The listing builds one solid part. Answer for the finished solid, in the listing's coordinates (mm). A direction names the side the tool comes from. Give positions to 0.01 mm unless a question says otherwise; leave off trailing zeros. Order: outer loops, then holes, each group sorted by start corner. A loop starts at its lowest first (then second) coordinate and runs counter-clockwise, first axis right, second up.
Autodesk Inventor part; units mm, degrees
ref_plane "YZ Plane" through (0, 0, 0) normal (1, 0, 0) x (0, 1, 0)
ref_plane "XZ Plane" through (0, 0, 0) normal (0, 1, 0) x (-1, 0, 0)
ref_plane "XY Plane" through (0, 0, 0) normal (0, 0, 1) x (1, 0, 0)
sketch "Sketch1" plane through (0, 0, 0) normal (0, 0, 1) x (1, 0, 0)
  line L0 (-33, 0) -> (33, 0)
  line L1 (33, 0) -> (33, -58)
  line L2 (33, -58) -> (-33, -58)
  line L3 (-33, -58) -> (-33, 0)
  point P0 (0, 0)
  dimension "d0" = 58
  dimension "d1" = 66
  dimension "d2" = 33
  dimension "d3" = 0
extrude "clamp_base" add sketch "Sketch1" against normal blind 190
sketch "Sketch2" plane through (0, 0, 0) normal (0, 0, 1) x (1, 0, 0)
  line L0 (-25, -58) -> (25, -58)
  line L1 (25, -58) -> (25, -8)
  line L2 (25, -8) -> (-25, -8)
  line L3 (-25, -8) -> (-25, -58)
  line L4 (-33, -58) -> (33, -58)
  point P0 (0, 0)
  dimension "d6" = 50
  dimension "d7" = 50
  dimension "d8" = 25
extrude "clamp_extrusion" cut sketch "Sketch2" against normal through all
sketch "Sketch4" plane through (-33, 0, 0) normal (0, 1, 0) x (1, 0, 0)
  line L0 (-35, 190) -> (101, 190)
  line L1 (101, 190) -> (101, 0)
  line L2 (101, 0) -> (-35, 0)
  line L3 (-35, 0) -> (-35, 190)
  line L4 (66, 0) -> (0, 0)
  line L5 (0, 190) -> (66, 190)
  line L6 (0, 0) -> (0, 190)
  line L7 (66, 0) -> (66, 190)
  point P0 (33, 0)
  dimension "d35" = 0
  dimension "d36" = 0
  dimension "d37" = 35
  dimension "d38" = 35
extrude "platform" add sketch "Sketch4" along normal blind 15
sketch "Sketch8" plane through (33, -58, 0) normal (1, 0, 0) x (0, 0, -1)
  line L0 (0, 0) -> (0, 58)
  line L1 (190, 58) -> (190, 0)
  point P0 (45, 24.0271)
  point P1 (145, 24.0271)
  dimension "d51" = 45
  dimension "d60" = 100
  dimension "d61" = 190
hole "clampHole" at (33, -33.9729, -45) at (33, -33.9729, -145) direction (-1, 0, 0) diameter 10 end through all
equation "\"d0\" = support_frame_squareBarDimension + support_baseClamp_thickness"
equation "\"d1\" = support_frame_squareBarDimension + 2 * support_baseClamp_thickness"
equation "\"d4\" = width"
equation "\"d6\" = support_frame_squareBarDimension"
equation "\"d7\" = support_frame_squareBarDimension"
equation "\"d37\" = support_baseClamp_platformLengthBuffer"
equation "\"d38\" = support_baseClamp_platformLengthBuffer"
equation "\"d13\" = support_baseClamp_platformThickness"
equation "\"d53\" = clampHoleDiameter"
equation "\"width\" = clampHoleDiameter + clampHoleSpacing + 2 * buffer"
equation "\"clampHoleSpacing\" = support_frame_clampHoleSpacing"
equation "\"clampHoleDiameter\" = support_frame_clampHoleDiameter"
equation "\"sleeveHoleDiameter\" = support_baseClamp_sleeveHoleDiameter"
equation "\"theta\" = hoop_angle_z"
equation "\"phi\" = support_baseClamp_sleeveSweepTerminationAngle"
equation "\"support_frame_squareBarDimension\" = 50"
equation "\"support_baseClamp_thickness\" = 8"
equation "\"support_baseClamp_sleeveHoleDiameter\" = 12"
equation "\"hoop_angle_z\" = 45deg"
equation "\"support_baseClamp_sleeveSweepTerminationAngle\" = 55deg"
equation "\"support_baseClamp_platformThickness\" = 15"
equation "\"support_baseClamp_platformWidthBuffer\" = 0"
equation "\"support_baseClamp_platformLengthBuffer\" = 35"
equation "\"rack_tooth_thickness\" = 5"
equation "\"rack_tooth_addendum\" = 5"
equation "\"rack_tooth_dedendum\" = 5"
equation "\"hoop_bearing_length\" = 5deg"
equation "\"hoop_cable_diam\" = 5"
equation "\"hoop_cable_pulley_diam\" = 22"
equation "\"secure_arm_radii\" = 9"
equation "\"secure_arm_hold_length\" = 35"
equation "\"secure_arm_angle\" = 20deg"
equation "\"support_frame_endHoleBuffer\" = 25"
equation "\"hoop_tabs_thickness\" = 6"
equation "\"support_frame_squareBarThickness\" = 5"
equation "\"wheelchair_deployed_length\" = 1067"
equation "\"wheelchair_deployed_height\" = 914"
equation "\"hoop_tabs_hole\" = 12"
equation "\"wheelchair_deployed_width\" = 635"
equation "\"support_frame_squareBarFillet\" = 2"
equation "\"sm_varx_pinPlate_thickness\" = 5"
equation "\"sm_varx_member_tolerance\" = 0.5"
equation "\"sm_varx_pinPlate_holeDiameter\" = 5"
equation "\"sm_varx_squareBarThickness\" = 2.5"
properties part number "support_basePart_nosleeve" material "Steel, High Strength, Low Alloy"
1) Given P1, Ø12, axis at x = 10, z = -65, coming from the -Y side; P2, Ø13, axis at y = -33.97, z = -45, coming from the -X side; P3, Ø9, axis at y = -33.97, z = -45, coming from the -X side; P4, Ø2, axis at x = -52.5, z = -64, coming from the -Y side, each flat-ended and moving along its own axis, determine where each tip first touches the part or whether it passes through.
Geometry says:
P1: stops at y = -8
P2: stops at x = -33
P3: passes through
P4: stops at y = 0
2) Find section A-A (y = -45.5). Write down the section's boundary in (x, z), then the cut area to 3 significant figures.
Geometry says:
outline: (-33, -190) - (-25, -190) - (-25, 0) - (-33, 0) - close; (25, -190) - (33, -190) - (33, 0) - (25, 0) - close
area: 3,040 mm2
3) Find section B-B (z = -45). Write down the section's boundary in (x, y).
Geometry says:
outline: (-68, 0) - (-33, 0) - (-33, -28.97) - (-25, -28.97) - (-25, -8) - (25, -8) - (25, -28.97) - (33, -28.97) - (33, 0) - (68, 0) - (68, 15) - (-68, 15) - close; (-33, -58) - (-25, -58) - (-25, -38.97) - (-33, -38.97) - close; (25, -58) - (33, -58) - (33, -38.97) - (25, -38.97) - close
4) Straight lines are drawn through the part: probe 1 along X at (y, z) = (-37, -162); probe 2 along Y at (x, z) = (29.25, -45); probe 3 along X at (y, z) = (-6, -139.5). For each, find the intervals that lie inside material, in ascending order.
Geometry says:
probe 1: x = -33 to -25, 25 to 33
probe 2: y = -58 to -38.97, -28.97 to 15
probe 3: x = -33 to 33
5) Find section C-C (z = -93). Write down the section's boundary in (x, y).
Geometry says:
outline: (-68, 0) - (-33, 0) - (-33, -58) - (-25, -58) - (-25, -8) - (25, -8) - (25, -58) - (33, -58) - (33, 0) - (68, 0) - (68, 15) - (-68, 15) - close
6) A tool of negligible diameter and unlimited length cuts with its end or side. For faces 5 (the flat face through (-1, 15, -96)), 6 (the flat face through (29, -58, -94)), 7 (the flat face through (50, 0, -96)), 8 (the flat face through (-25, -33, -94)), 9 (the flat face through (-51, 0, -96)), from which of +Z, -Z, +X, -X, +Y, -Y can it reach the whole face along a straight path? Write none if from no direction.
Geometry says:
face 5: +Z, -Z, +X, -X, +Y
face 6: +Z, -Z, +X, -X, -Y
face 7: +Z, -Z, +X, -Y
face 8: +Z, -Z, -Y
face 9: +Z, -Z, -X, -Y
7) For a pull along X with two mould halves and no side action, classify faces 1 (the flat face through (-33, -29, -94)), 2 (the flat face through (33, -29, -94)), 3 (the flat face through (-1, -6, -190)), 4 (the flat face through (25, -33, -94)) as +X half, -X half, draft (parallel to the pull), parting line (faces both ways), or undercut.
Geometry says:
face 1: -X half
face 2: +X half
face 3: draft
face 4: undercut
8) Find section D-D (x = -9). Write down the section's boundary in (y, z), then the cut area to 3 significant figures.
Geometry says:
outline: (-8, -190) - (15, -190) - (15, 0) - (-8, 0) - close
area: 4,370 mm2
